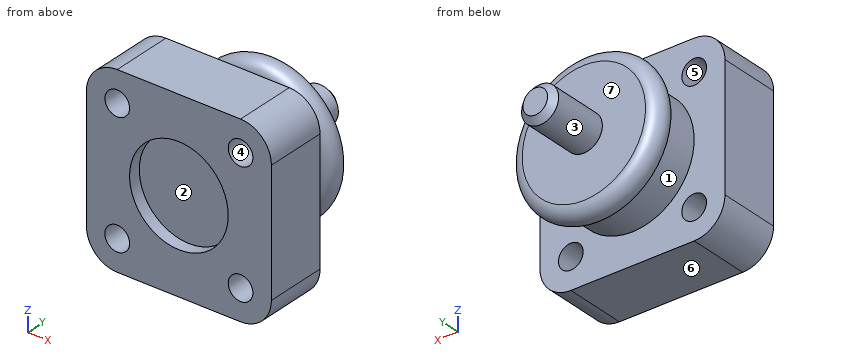
```python
from build123d import *

# Parameters (mm, degrees)
SKETCH1_R           = 2
BOSS_EXTRUDE1_DEPTH = 10
SKETCH2_R           = 10
BOSS_EXTRUDE2_DEPTH = 10
SKETCH3_R           = 2
SKETCH4_R           = 3
BOSS_EXTRUDE3_DEPTH = 10
CHAMFER1_SIZE       = 1
SKETCH5_R           = 8
CUT_EXTRUDE1_DEPTH  = 2


with BuildPart() as part:
    # Sketch1 → Boss-Extrude1 (new body)
    with BuildSketch(Plane(origin=(0, 0, 0), x_dir=(1, 0, 0), z_dir=(0, 1, 0))):
        with BuildLine():
            Line((-10, -15), (10, -15))
            ThreePointArc((10, -15), (13.535533906, -13.535533906), (15, -10))
            Line((15, -10), (15, 10))
            ThreePointArc((15, 10), (13.535533906, 13.535533906), (10, 15))
            Line((10, 15), (-10, 15))
            ThreePointArc((-10, 15), (-13.535533906, 13.535533906), (-15, 10))
            Line((-15, 10), (-15, -10))
            ThreePointArc((-15, -10), (-13.535533906, -13.535533906), (-10, -15))
        make_face()
        with Locations(Location((-10, 10, 0), (0, 0, 270))):
            Circle(SKETCH1_R, mode=Mode.SUBTRACT)
        with Locations(Location((10, 10, 0), (0, 0, 270))):
            Circle(SKETCH1_R, mode=Mode.SUBTRACT)
        with Locations(Location((-10, -10, 0), (0, 0, 270))):
            Circle(SKETCH1_R, mode=Mode.SUBTRACT)
        with Locations(Location((10, -10, 0), (0, 0, 270))):
            Circle(SKETCH1_R, mode=Mode.SUBTRACT)
    extrude(amount=BOSS_EXTRUDE1_DEPTH)

    # Sketch2 → Boss-Extrude2 (add)
    with BuildSketch(Plane(origin=(0, 10, 0), x_dir=(1, 0, 0), z_dir=(0, 1, 0))):
        with Locations(Location((0, 0, 0), (0, 0, 270))):
            Circle(SKETCH2_R)
    extrude(amount=BOSS_EXTRUDE2_DEPTH)

    # Sketch3 → Revolve1 (revolve)
    with BuildSketch(Plane(origin=(0, 0, 0), x_dir=(0, 0, -1), z_dir=(1, 0, 0))):
        with Locations((-10, 18)):
            Circle(SKETCH3_R)
    revolve(axis=Axis((0, 0, 0), (0, 1, 0)))

    # Sketch4 → Boss-Extrude3 (add)
    with BuildSketch(Plane(origin=(0, 20, 0), x_dir=(1, 0, 0), z_dir=(0, 1, 0))):
        with Locations(Location((0, 0, 0), (0, 0, 270))):
            Circle(SKETCH4_R)
    extrude(amount=BOSS_EXTRUDE3_DEPTH)

    # Chamfer1
    chamfer1_edges = [part.edges().sort_by_distance(p)[0] for p in [
        (0, 30, -3),
    ]]
    chamfer(chamfer1_edges, length=CHAMFER1_SIZE)

    # Sketch5 → Cut-Extrude1 (cut)
    with BuildSketch(Plane.XZ):
        with Locations(Location((0, 0, 0), (0, 0, 270))):
            Circle(SKETCH5_R)
    extrude(amount=-CUT_EXTRUDE1_DEPTH, mode=Mode.SUBTRACT)


solid = part.part
```
Geometry check sheet. Reference: the model listing, model coordinates, mm. Face numbers are marked on the shaded views. A direction names the side the tool comes from. Coordinates: 2 decimals unless noted, no trailing zeros. Order: outer loops, then holes, each group sorted by start corner. A loop starts at its lowest first (then second) coordinate and runs counter-clockwise, first axis right, second up.
Item 1: Section check B-B (y = 25.5). Enter the section's corners in (x, z).
Item 2: Depth check by flat-ended pin: pin 1 (10 mm diameter, centred on x = 6.5, z = -5, fed in from +Y); pin 2 (10 mm diameter, centred on x = 5.5, z = -5, fed in from +Y); pin 3 (10 mm diameter, centred on x = 2.5, z = 1.5, fed in from -Y). Enter the tip coordinate at first touch or a pass-through.
Item 3: Mould release check, pull along Z, two halves, no side actions. Record for the marked faces 4, 5, 6 and 7: released by +Z, released by -Z, zero draft, split by the parting line, or undercut.
Item 4: Tool access check on the marked faces 1, 2 and 3. Record the directions out of +Z, -Z, +X, -X, +Y, -Y that give a thin tool (end or side, any length) a straight path to the whole face; none if there is none.
Item 5: Section check A-A (z = 0). Enter the section's corners in (x, y), plus the area to 3 significant figures.
Item 6: Scan lines: line 1 along X through (y, z) = (2.75, -10); line 2 along Y through (x, z) = (-11, 7.5); line 3 along Z through (x, y) = (-9, 7.25). Record each from-to range of solid material in increasing order.
Check sheet entries:
1. outline: circle Ø6 at (0, 0)
2. pin 1: stops at y = 20
2. pin 2: stops at y = 29.57
2. pin 3: stops at y = 2
3. face 4: undercut
3. face 5: undercut
3. face 6: released by -Z
3. face 7: zero draft
4. face 1: none
4. face 2: -Y
4. face 3: +Y
5. outline: (-15, 0) - (-8, 0) - (-8, 2) - (8, 2) - (8, 0) - (15, 0) - (15, 10) - (10, 10) - (10, 16) arc R2 ccw to (10, 20) - (3, 20) - (3, 29) - (2, 30) - (-2, 30) - (-3, 29) - (-3, 20) - (-10, 20) arc R2 ccw to (-10, 16) - (-10, 10) - (-15, 10) - close
5. area: 540 mm2
6. line 1: x = -15 to -12, -8 to 8, 12 to 15
6. line 2: y = 0 to 10
6. line 3: z = -15 to -11.73, -8.27 to 8.27, 11.73 to 15
